from build123d import *

# Parameters (mm, degrees)
SKETCH1_R           = 1.5
BOSS_EXTRUDE1_DEPTH = 4


with BuildPart() as part:
    # Sketch1 → Boss-Extrude1 (new body)
    with BuildSketch(Plane.XY):
        with BuildLine():
            Line((-3, 0), (-45, 0))
            ThreePointArc((-45, 0), (-47.121320344, 0.878679656), (-48, 3))
            Line((-48, 3), (-48, 68))
            ThreePointArc((-48, 68), (-47.121320344, 70.121320344), (-45, 71))
            Line((-45, 71), (54, 71))
            ThreePointArc((54, 71), (56.121320344, 71.878679656), (57, 74))
            Line((57, 74), (57, 78))
            ThreePointArc((57, 78), (56.121320344, 80.121320344), (54, 81))
            Line((54, 81), (-55, 81))
            ThreePointArc((-55, 81), (-57.121320344, 80.121320344), (-58, 78))
            Line((-58, 78), (-58, -7))
            ThreePointArc((-58, -7), (-57.121320344, -9.121320344), (-55, -10))
            Line((-55, -10), (-3, -10))
            ThreePointArc((-3, -10), (-0.878679656, -9.121320344), (0, -7))
            Line((0, -7), (0, -3))
            ThreePointArc((0, -3), (-0.878679656, -0.878679656), (-3, 0))
        make_face()
        with Locations((-5, -5)):
            Circle(SKETCH1_R, mode=Mode.SUBTRACT)
    extrude(amount=BOSS_EXTRUDE1_DEPTH)


solid = part.part
For this review, take the finished solid that the model builds, in its own axes (mm). A direction names the side the tool comes from. Give positions to 0.01 mm unless a question says otherwise; leave off trailing zeros. Order: outer loops, then holes, each group sorted by start corner. A loop starts at its lowest first (then second) coordinate and runs counter-clockwise, first axis right, second up. Notation, with made-up numbers: M -29,-36.75 L 6,-36.75 A36 ccw 6,-1.75 Z; hole C 18.5,72.5 d5. An arc over 180 degrees is marked long. Answer in a Markdown table with one row per item. Add a question column.
(1) Wall thickness on probe 1 along Y at (x, z) = (-5, 1.4); probe 2 along Y at (x, z) = (-35, 0.85); probe 3 along Y at (x, z) = (50.5, 0.65): over which ranges is each line inside the solid? List them lowest first. Write a range as [from, to].
(2) Consider section C-C on y = -5. State the section outline as (x, z) points, and give its area (3 significant figures).
(3) For faces 1 (the face through (0, -5, 2)), 2 (the face through (-6.11, -3.99, 1.97)), 3 (the face through (-24, 0, 2)), list the 3-axis set-ups (+Z, -Z, +X, -X, +Y, -Y) from which the entire face can be reached by the end or side of a thin tool; tool diameter is ignored.
(4) For pin 1 (3.5 mm diameter, centred on x = -5, y = -5, fed in from +Z), flat-tipped, find the tip position at first contact; note if it passes through.
(5) Consider section A-A on x = -5. State the section outline as (y, z) points.
(6) Consider section D-D on x = -40. State the section outline as (y, z) points, and give its area (3 significant figures).
(7) Mouldability with a two-part tool opening along Y and no side actions: class faces 4 (the face through (-58, 36, 2)), 5 (the face through (-47.14, 70.1, 1.97)), 6 (the face through (-57.14, -9.1, 1.97)) as +Y half, -Y half, draft (parallel to the pull), parting line (faces both ways), or undercut.
(8) Consider section B-B on z = 3.2. State the section outline as (x, y) points.
Evaluation:
| question | item | result |
|---|---|---|
| 1 | probe 1 | y = [-10, -6.5], [-3.5, 0], [71, 81] |
| 1 | probe 2 | y = [-10, 0], [71, 81] |
| 1 | probe 3 | y = [71, 81] |
| 2 | outline | M -58,0 L -6.5,0 L -6.5,4 L -58,4 Z; M -3.5,0 L 0,0 L 0,4 L -3.5,4 Z |
| 2 | area | 220 mm^2 |
| 3 | face 1 | +Z, -Z, +X, -Y |
| 3 | face 2 | +Z, -Z |
| 3 | face 3 | +Z, -Z, +X |
| 4 | pin 1 | stops at z = 4 |
| 5 | outline | M -10,0 L -6.5,0 L -6.5,4 L -10,4 Z; M -3.5,0 L 0,0 L 0,4 L -3.5,4 Z; M 71,0 L 81,0 L 81,4 L 71,4 Z |
| 6 | outline | M -10,0 L 0,0 L 0,4 L -10,4 Z; M 71,0 L 81,0 L 81,4 L 71,4 Z |
| 6 | area | 80.0 mm^2 |
| 7 | face 4 | draft |
| 7 | face 5 | undercut |
| 7 | face 6 | -Y half |
| 8 | outline | M -58,-7 A3 ccw -55,-10 L -3,-10 A3 ccw 0,-7 L 0,-3 A3 ccw -3,0 L -45,0 A3 cw -48,3 L -48,68 A3 cw -45,71 L 54,71 A3 ccw 57,74 L 57,78 A3 ccw 54,81 L -55,81 A3 ccw -58,78 Z; hole C -5,-5 d3 |
